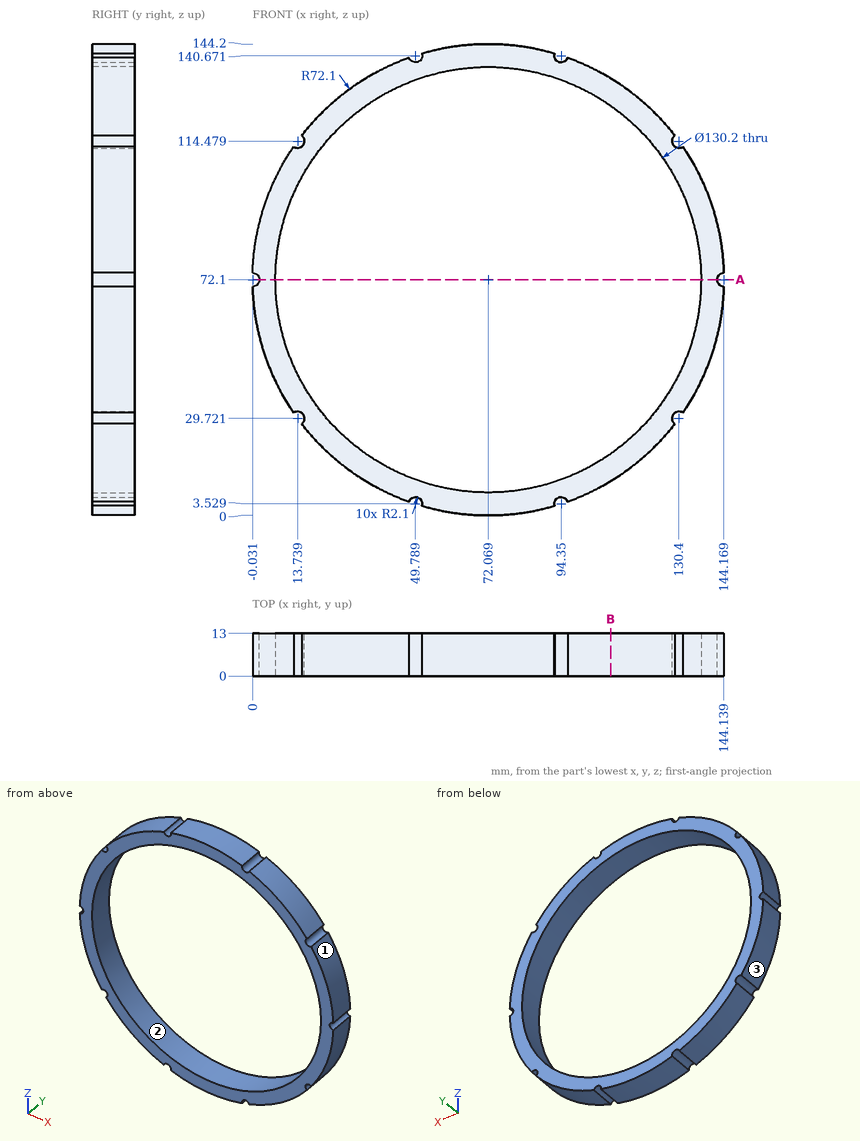
Print and shaded views of the part. All mm, measured from the part's lowest x, y and z. Coordinates: 2 decimals unless noted, no trailing zeros. Order: outer loops, then holes, each group sorted by start corner. A loop starts at its lowest first (then second) coordinate and runs counter-clockwise, first axis right, second up. Notation, with made-up numbers: (48, 55) -> (56, 55) arc R29 ccw to (56, 89) -> close; hole circle Ø6 at (10, 2). An arc over 180 degrees is marked (long way). Use one line per item in the form item = value. Start each with the question number.
1) Drop flat-ended pins along their axis: pin 1 (3 mm diameter, centred on y = 10, z = 87, fed in from +X); pin 2 (3 mm diameter, centred on y = 1.5, z = 50.5, fed in from +X); pin 3 (2 mm diameter, centred on x = 84.5, y = 8.5, fed in from -Z). Give the stop position or say it passes through.
2) Band-saw the part on A-A on z = 72.1. Give the cut face in (x, y), then the cut area to 3 significant figures.
3) Pull direction Z, two halves, no side cores. Call the marked faces 1, 2 and 3: +Z half, -Z half, draft (parallel to the pull), parting line (faces both ways), or undercut.
4) Drill centre lines: L1, parallel to Z at x = 111, y = 9.75 (1 decimal); L2, parallel to Z at x = 88, y = 4.25; L3, parallel to X at y = 2, z = 109.5 (1 decimal). Where is each one in solid material? Low to high. Write a range as [from, to].
5) Band-saw the part on B-B on x = 109.5. Give the cut face in (y, z), then the cut area to 3 significant figures.
Entries:
q1.pin_1 = 142.91
q1.pin_2 = 141.31
q1.pin_3 = 0.91
q2.outline = (2.07, 0) -> (6.97, 0) -> (6.97, 13) -> (2.07, 13) -> close; (137.17, 0) -> (142.07, 0) -> (142.07, 13) -> (137.17, 13) -> close
q2.area = 127 mm2
q3.face_1 = +Z half
q3.face_2 = undercut
q3.face_3 = -Z half
q4.L1 = [11.4, 19.9], [124.3, 132.8]
q4.L2 = [1.78, 8.98], [135.22, 142.42]
q4.L3 = [10.4, 18.8], [125.4, 133.7]
q5.outline = (0, 10.48) -> (13, 10.48) -> (13, 18.84) -> (0, 18.84) -> close; (0, 125.36) -> (13, 125.36) -> (13, 133.72) -> (0, 133.72) -> close
q5.area = 217 mm2
